Model file for the job. Use its own axes, mm. A direction names the side the tool comes from. Coordinates: 2 decimals unless noted, no trailing zeros. Write each loop counter-clockwise with the first axis right and the second up, starting at its lowest first coordinate (ties: lowest second). Pieces come first, ordered by that corner, then holes. Notation, with made-up numbers: M -20.5,47.5 L 34.5,47.5 A32 cw 34.5,83.5 Z; hole C -36.75,59 d7. An arc over 180 degrees is marked long. One line per question, with ' | ' between items. Start each with the question number.
(1) Two-plate mould, pull along X, no slides. Class faces 1 (the face through (0, 1, 3.25)), 2 (the face through (-1, 1, -4.25)), 3 (the face through (-4.25, 1, 0)): +X half, -X half, draft (parallel to the pull), parting line (faces both ways), or undercut.
(2) Tool access for faces 4 (the face through (0, 1, 4.25)), 5 (the face through (3.25, 1, 0)): list every direction of +Z, -Z, +X, -X, +Y, -Y with a clear straight run to the whole face (end or side of a thin tool).
(3) Wall check: probe 1 along X at (y, z) = (-56.5, -0.5); probe 2 along Y at (x, z) = (1, -3.5). Give the ranges that are in metal, low to high.
(4) Cut at C-C (y = 21.5). Write the cut outline in (x, z), plus the area to 3 significant figures.
from build123d import *

# Parameters (mm, degrees)
SKETCH1_W           = 8.5
SKETCH1_H           = 8.5
SKETCH1_W_2         = 6.5
SKETCH1_H_2         = 6.5
BOSS_EXTRUDE1_DEPTH = 85.1
FILLET1_R           = 1
FILLET2_R           = 1
FILLET3_R           = 1


with BuildPart() as part:
    # Sketch1 → Boss-Extrude1 (new, symmetric)
    with BuildSketch(Plane(origin=(0, 0, 0), x_dir=(1, 0, 0), z_dir=(0, 1, 0))):
        Rectangle(SKETCH1_W, SKETCH1_H)
        Rectangle(SKETCH1_W_2, SKETCH1_H_2, mode=Mode.SUBTRACT)
    extrude(amount=BOSS_EXTRUDE1_DEPTH, both=True)

    # Fillet1
    fillet1_edges = [part.edges().sort_by_distance(p)[0] for p in [
        (4.25, 0, -4.25),
    ]]
    fillet(fillet1_edges, radius=FILLET1_R)

    # Fillet2
    fillet2_edges = [part.edges().sort_by_distance(p)[0] for p in [
        (-4.25, 85.1, 0),
        (0, 85.1, 4.25),
        (-0.5, 85.1, -4.25),
        (3.957106781, 85.1, -3.957106781),
        (4.25, 85.1, 0.5),
    ]]
    fillet(fillet2_edges, radius=FILLET2_R - 0.0001)  # a hair under: the kernel refuses the full size

    # Fillet3
    fillet3_edges = [part.edges().sort_by_distance(p)[0] for p in [
        (-0.5, -85.1, -4.25),
        (3.957106781, -85.1, -3.957106781),
        (0, -85.1, 4.25),
        (-4.25, -85.1, 0),
        (4.25, -85.1, 0.5),
    ]]
    fillet(fillet3_edges, radius=FILLET3_R - 0.0001)  # a hair under: the kernel refuses the full size


solid = part.part
Filled in:
1) face 1: undercut | face 2: draft | face 3: -X half
2) face 4: +Z, +X, -X, +Y, -Y | face 5: +Y, -Y
3) probe 1: -4.25 to -3.25, 3.25 to 4.25 | probe 2: -85.07 to 85.07
4) outline: M -4.25,-4.25 L 3.25,-4.25 A1 ccw 4.25,-3.25 L 4.25,4.25 L -4.25,4.25 Z; hole M -3.25,-3.25 L 3.25,-3.25 L 3.25,3.25 L -3.25,3.25 Z | area: 29.8 mm²
